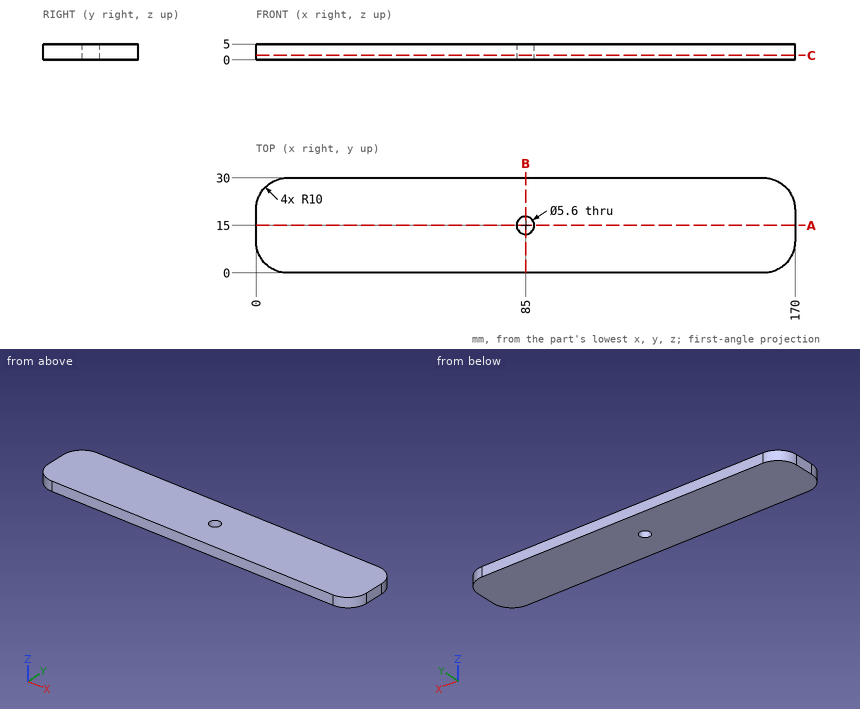
Part print with two shaded views. Sizes in mm from the minimum x, y, z corner. Give positions to 0.01 mm unless a question says otherwise; leave off trailing zeros. Order: outer loops, then holes, each group sorted by start corner. A loop starts at its lowest first (then second) coordinate and runs counter-clockwise, first axis right, second up. Notation, with made-up numbers: M 1.25,71 L 59.25,71 A14 cw 59.25,94 Z; hole C -19,-17.75 d10. An arc over 180 degrees is marked long. Use one line per item in the form item = value.
1) Drop flat-ended pins along their axis: pin 1 (3 mm diameter, centred on y = 21.5, z = 1, fed in from -X); pin 2 (3 mm diameter, centred on y = 6, z = 1.5, fed in from +X). Give the stop position or say it passes through.
Calculated:
pin_1 = 0
pin_2 = 169.68
2) Saw through at B-B (x = 85). Give the cut face in (y, z), plus the area to 3 significant figures.
Calculated:
outline = M 0,0 L 12.2,0 L 12.2,5 L 0,5 Z; M 17.8,0 L 30,0 L 30,5 L 17.8,5 Z
area = 122 mm2
3) Saw through at A-A (y = 15). Give the cut face in (x, z).
Calculated:
outline = M 0,0 L 82.2,0 L 82.2,5 L 0,5 Z; M 87.8,0 L 170,0 L 170,5 L 87.8,5 Z
4) Probe probe 1 along Y at (x, z) = (85, 3.65); probe 2 along X at (y, z) = (20.75, 2.15); probe 3 along X at (y, z) = (15.75, 1.7). List the from-to ranges inside material, lowest first.
Calculated:
probe_1 = 0 to 12.2, 17.8 to 30
probe_2 = 0.03 to 169.97
probe_3 = 0 to 82.3, 87.7 to 170
5) Saw through at C-C (z = 1.4). Give the cut face in (x, y), plus the area to 3 significant figures.
Calculated:
outline = M 0,10 A10 ccw 10,0 L 160,0 A10 ccw 170,10 L 170,20 A10 ccw 160,30 L 10,30 A10 ccw 0,20 Z; hole C 85,15 d5.6
area = 4,990 mm2
